Build history of the part. All positions in model axes, mm. Face numbers are marked on the shaded views. Round coordinates to 2 decimals unless told otherwise and drop trailing zeros. Write each loop counter-clockwise with the first axis right and the second up, starting at its lowest first coordinate (ties: lowest second). Pieces come first, ordered by that corner, then holes. Notation, with made-up numbers: M -22,84.5 L -16,84.5 A25 cw -16,98.5 Z; hole C 54,43 d2. An arc over 180 degrees is marked long. Use a Markdown table: item, result.
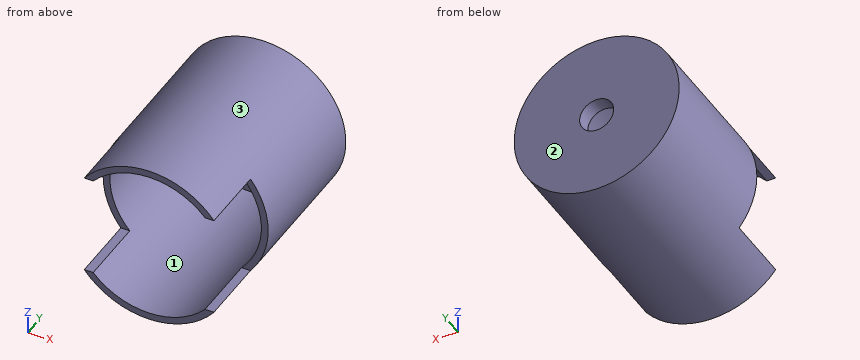
from build123d import *

# Parameters (mm, degrees)
SKETCH_1_R               = 9.7
EXTRUDE_1_DEPTH          = 25
SKETCH_5_R               = 8.9
CUT_EXTRUDE_2_DEPTH      = 23
CUT_EXTRUDE_3_DEPTH      = 29.516311122
CUT_EXTRUDE_3_DEPTH_BACK = 29.516311122
SKETCH_6_W               = 12
SKETCH_6_H               = 16
SKETCH_9_R               = 2
CUT_EXTRUDE_4_DEPTH      = 29.516311122
CHAMFER_5_SIZE           = 0.2


with BuildPart() as part:
    # Sketch 1 → Extrude 1 (new body)
    with BuildSketch(Plane(origin=(0, 0, 0), x_dir=(1, 0, 0), z_dir=(0, 1, 0))):
        with Locations(Location((0, 0, 0), (0, 0, 270))):
            Circle(SKETCH_1_R)
    extrude(amount=EXTRUDE_1_DEPTH)

    # Sketch 5 → Cut-Extrude 2 (cut)
    with BuildSketch(Plane.XZ):
        with Locations(Location((0, 0, 0), (0, 0, 270))):
            Circle(SKETCH_5_R)
    extrude(amount=-CUT_EXTRUDE_2_DEPTH, mode=Mode.SUBTRACT)

    # Sketch 6 → Cut-Extrude 3 (cut, two sides: drawn at the far end of the back side and taken through both)
    with BuildSketch(Plane(origin=(0, 0, 0), x_dir=(0, 0, -1), z_dir=(1, 0, 0)).offset(-CUT_EXTRUDE_3_DEPTH_BACK)):
        Rectangle(SKETCH_6_W, SKETCH_6_H)
    extrude(amount=CUT_EXTRUDE_3_DEPTH + CUT_EXTRUDE_3_DEPTH_BACK, mode=Mode.SUBTRACT)

    # Sketch 9 → Cut-Extrude 4 (cut, through all)
    with BuildSketch(Plane(origin=(0, 25, 0), x_dir=(1, 0, 0), z_dir=(0, 1, 0))):
        with Locations(Location((0, 0, 0), (0, 0, 270))):
            Circle(SKETCH_9_R)
    extrude(amount=-CUT_EXTRUDE_4_DEPTH, mode=Mode.SUBTRACT)

    # Chamfer 5
    chamfer_5_edges = [part.edges().sort_by_distance(p)[0] for p in [
        (0, 23, -2),
    ]]
    chamfer(chamfer_5_edges, length=CHAMFER_5_SIZE)


solid = part.part
Q1. Cut at C-C on z = 4.25. Give the cut face in (x, y), and give its area (3 significant figures).
Response values:
| item | result |
|---|---|
| outline | M -8.72,8 L -7.82,8 L -7.82,23 L 7.82,23 L 7.82,8 L 8.72,8 L 8.72,25 L -8.72,25 Z |
| area | 61.9 mm2 |
Q2. Cut at A-A on x = 0. Give the cut face in (y, z), and give its area (3 significant figures).
Response values:
| item | result |
|---|---|
| outline | M 0,-9.7 L 25,-9.7 L 25,-2 L 23.2,-2 L 23,-2.2 L 23,-8.9 L 0,-8.9 Z; M 0,8.9 L 23,8.9 L 23,2.2 L 23.2,2 L 25,2 L 25,9.7 L 0,9.7 Z |
| area | 67.6 mm2 |
Q3. Cut at B-B on z = 0. Give the cut face in (x, y).
Response values:
| item | result |
|---|---|
| outline | M -9.7,8 L -8.9,8 L -8.9,23 L -2.2,23 L -2,23.2 L -2,25 L -9.7,25 Z; M 2,23.2 L 2.2,23 L 8.9,23 L 8.9,8 L 9.7,8 L 9.7,25 L 2,25 Z |
Q4. Drill centre lines: L1, parallel to X at y = 24.3, z = 0; L2, parallel to Y at x = 3.5, z = -3; L3, parallel to Z at x = -3, y = 6.75. Where is each one in solid material? Low to high.
Response values:
| item | result |
|---|---|
| L1 | x = -9.7 to -2, 2 to 9.7 |
| L2 | y = 23 to 25 |
| L3 | z = -9.22 to -8.38, 8.38 to 9.22 |
Q5. Drop flat-ended pins along their axis: P1, Ø1.5, axis at x = -1, y = 15, coming from the -Z side; P2, Ø1.6, axis at x = 8.5, z = 0.5, coming from the -Y side; P3, Ø0.8, axis at x = 7, y = 3.5, coming from the -Z side. Give the stop position or say it passes through.
Response values:
| item | result |
|---|---|
| P1 | stops at z = -9.7 |
| P2 | stops at y = 8 |
| P3 | stops at z = -7.11 |
Q6. Two-plate mould, pull along Z, no slides. Class the marked faces 1, 2 and 3: +Z half, -Z half, draft (parallel to the pull), parting line (faces both ways), or undercut.
Response values:
| item | result |
|---|---|
| face 1 | undercut |
| face 2 | draft |
| face 3 | parting line |
Q7. Cut at D-D on y = 13.5. Give the cut face in (x, z), and give its area (3 significant figures).
Response values:
| item | result |
|---|---|
| outline | C 0,0 d19.4; hole C 0,0 d17.8 |
| area | 46.7 mm2 |
